Build history of the part. All positions in model axes, mm. A direction names the side the tool comes from. Coordinates: 2 decimals unless noted, no trailing zeros. Write each loop counter-clockwise with the first axis right and the second up, starting at its lowest first coordinate (ties: lowest second). Pieces come first, ordered by that corner, then holes.
```python
from build123d import *

# Parameters (mm, degrees)
F0_W     = 304.8
F0_H     = 152.4
F1_DEPTH = 152.4
F2_W     = 292.1
F2_H     = 292.1
F3_DEPTH = 139.7
F5_DEPTH = 12.7
F4_W     = 38.1
F4_H     = 19.05
F6_DEPTH = 12.7


with BuildPart() as f1:
    # F0 (on Front) → F1 (new body, symmetric)
    with BuildSketch(Plane.XZ):
        with Locations((3.97213, -16.929825)):
            Rectangle(F0_W, F0_H)
    extrude(amount=F1_DEPTH, both=True)

    # F2 (on face) → F3 (cut)
    with BuildSketch(Plane(origin=(0, 0, -93.129825), x_dir=(1, 0, 0), z_dir=(0, 0, -1))):
        with Locations((3.97213, 0)):
            Rectangle(F2_W, F2_H)
    extrude(amount=-F3_DEPTH, mode=Mode.SUBTRACT)

    # F4 (on face) → F5 (cut)
    with BuildSketch(Plane.XY.offset(59.270175)):
        Polygon((3.97213, 0), (3.97213, 146.05), (-142.07787, 146.05), (-142.07787, -146.05), (3.97213, -146.05), align=None)
    extrude(amount=-F5_DEPTH, mode=Mode.SUBTRACT)

    # F4 (on face) → F6 (join)
    with BuildSketch(Plane.XY.offset(59.270175)):
        with Locations((80.17213, 9.525)):
            Rectangle(F4_W, F4_H)
        with Locations((80.17213, -9.525)):
            Rectangle(F4_W, F4_H)
    extrude(amount=F6_DEPTH)


solid = f1.part
```
1. Flat gauge pins, fed straight in: pin 1 (4 mm diameter, centred on y = -7.5, z = 64, fed in from +X); pin 2 (3 mm diameter, centred on x = 17.5, y = 44, fed in from +Z); pin 3 (6.5 mm diameter, centred on x = 78.5, z = 63.5, fed in from +Y). Where does each tip first touch, or does it go through?
Computed values:
pin 1: stops at x = 99.22
pin 2: stops at z = 59.27
pin 3: stops at y = 19.05
2. 3-axis set-ups, long thin cutter, end or side, ignore diameter. For faces 1 (the face through (3.972, -2, 53)), 2 (the face through (61.122, 0, 66)), 3 (the face through (80, -19.05, 66)): which of +Z, -Z, +X, -X, +Y, -Y reach the whole face in a straight line?
Computed values:
face 1: +Z, -Z
face 2: +Z, -X, +Y, -Y
face 3: +Z, +X, -X, -Y
3. Saw through at C-C on y = 44. List the corners of the cut face in (x, z), plus the area to 3 significant figures.
Computed values:
outline: (-148.43, -93.13) - (-142.08, -93.13) - (-142.08, 59.27) - (-148.43, 59.27) - close; (3.97, 46.57) - (150.02, 46.57) - (150.02, -93.13) - (156.37, -93.13) - (156.37, 59.27) - (3.97, 59.27) - close
area: 3,790 mm2
4. Mould opens along X. For faces 4 (the face through (99.222, 0, 66)), 5 (the face through (2, -146.05, -18)), 6 (the face through (2, 152.4, -16)) say: +X half, -X half, draft (parallel to the pull), parting line (faces both ways), or undercut.
Computed values:
face 4: +X half
face 5: undercut
face 6: draft
5. Saw through at A-A on x = -51.5. List the corners of the cut face in (y, z), plus the area to 3 significant figures.
Computed values:
outline: (-152.4, -93.13) - (-146.05, -93.13) - (-146.05, 59.27) - (-152.4, 59.27) - close; (146.05, -93.13) - (152.4, -93.13) - (152.4, 59.27) - (146.05, 59.27) - close
area: 1,940 mm2
6. Saw through at B-B on z = -35. List the corners of the cut face in (x, y), plus the area to 3 significant figures.
Computed values:
outline: (-148.43, -152.4) - (156.37, -152.4) - (156.37, 152.4) - (-148.43, 152.4) - close; hole (-142.08, -146.05) - (150.02, -146.05) - (150.02, 146.05) - (-142.08, 146.05) - close
area: 7,580 mm2
7. Saw through at D-D on x = 105. List the corners of the cut face in (y, z), plus the area to 3 significant figures.
Computed values:
outline: (-152.4, -93.13) - (-146.05, -93.13) - (-146.05, 46.57) - (146.05, 46.57) - (146.05, -93.13) - (152.4, -93.13) - (152.4, 59.27) - (-152.4, 59.27) - close
area: 5,650 mm2
8. Probe line 1 along X through (y, z) = (-65, -59); line 2 along Y through (x, z) = (-61, -53.5); line 3 along X through (y, z) = (54.5, 59). List the from-to ranges inside material, lowest first.
Computed values:
line 1: x = -148.43 to -142.08, 150.02 to 156.37
line 2: y = -152.4 to -146.05, 146.05 to 152.4
line 3: x = -148.43 to -142.08, 3.97 to 156.37
